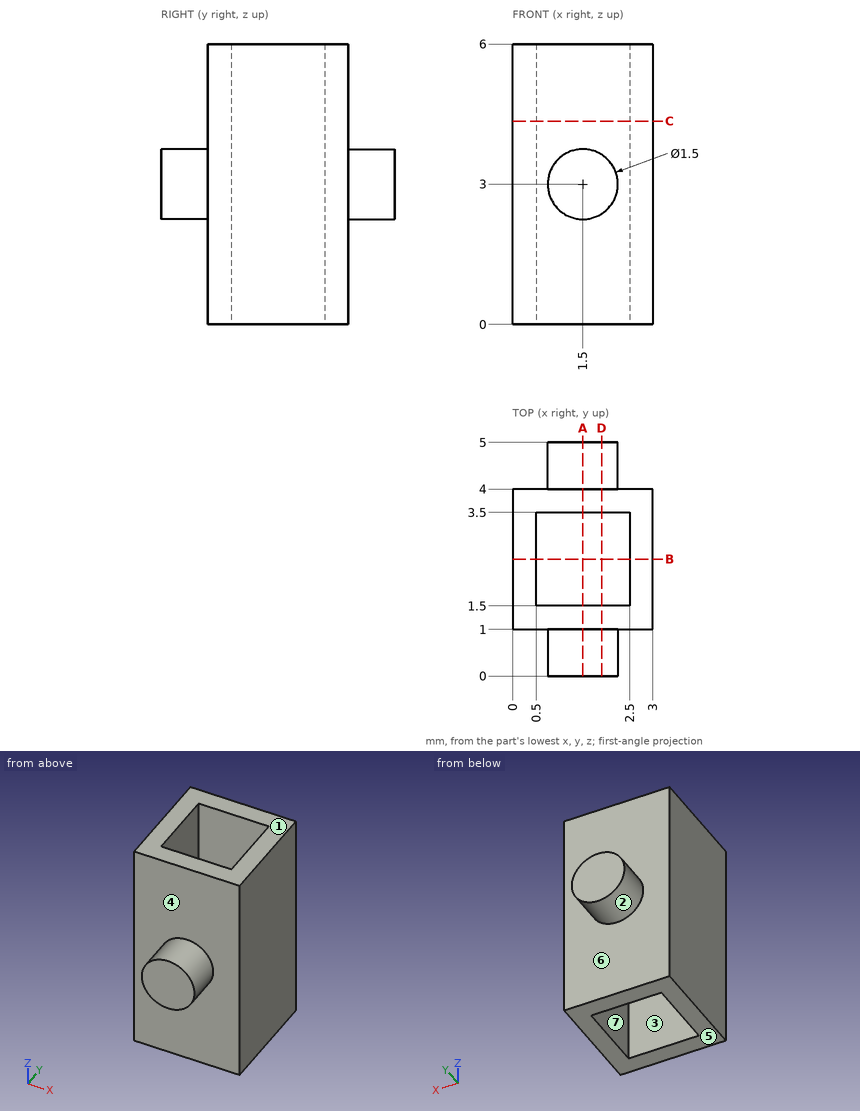
Geometry check sheet. Reference: drawing and pictorial views, mm from the part's lowest x, y, z. A direction names the side the tool comes from. Round coordinates to 2 decimals unless told otherwise and drop trailing zeros. Loops run counter-clockwise (first coordinate to the right, second up) from the corner with the lowest first, then second, coordinate; pieces in that order, holes last. Notation, with made-up numbers: (74.25, -25) - (91.25, -25) arc R19 cw to (91.25, -5) - close; hole circle Ø3 at (82, 44). An arc over 180 degrees is marked (long way). Use a Markdown table: item, result. Add a question column.
1. Section check C-C, the plane z = 4.35. Record the boundary of the cut face in (x, y), plus the area to 3 significant figures.
2. Thickness scan on probe 1 along Y at (x, z) = (1.9, 5.05); probe 2 along X at (y, z) = (3.15, 1.9); probe 3 along Y at (x, z) = (2.8, 2.9). Record the ranges inside material, lowest first. Write a range as [from, to].
3. Access from +Z, -Z, +X, -X, +Y, -Y to the whole of each face (thin tool, end or side, straight path). Record for the marked faces 1, 2, 3 and 4.
4. Section check D-D, the plane x = 1.9. Record the boundary of the cut face in (y, z).
5. Section check A-A, the plane x = 1.5. Record the boundary of the cut face in (y, z).
6. Release check for a two-part mould opening along Y. For the marked faces 5, 6 and 7 record: released by +Y, released by -Y, zero draft, split by the parting line, or undercut.
7. Section check B-B, the plane y = 2.5. Record the boundary of the cut face in (x, z).
Checks:
| question | item | result |
|---|---|---|
| 1 | outline | (0, 1) - (3, 1) - (3, 4) - (0, 4) - close; hole (0.5, 1.5) - (2.5, 1.5) - (2.5, 3.5) - (0.5, 3.5) - close |
| 1 | area | 5.00 mm^2 |
| 2 | probe 1 | y = [1, 1.5], [3.5, 4] |
| 2 | probe 2 | x = [0, 0.5], [2.5, 3] |
| 2 | probe 3 | y = [1, 4] |
| 3 | face 1 | +Z, +X, -X, +Y, -Y |
| 3 | face 2 | +Y |
| 3 | face 3 | +Z, -Z |
| 3 | face 4 | -Y |
| 4 | outline | (0, 2.37) - (1, 2.37) - (1, 0) - (1.5, 0) - (1.5, 6) - (1, 6) - (1, 3.63) - (0, 3.63) - close; (3.5, 0) - (4, 0) - (4, 2.37) - (5, 2.37) - (5, 3.63) - (4, 3.63) - (4, 6) - (3.5, 6) - close |
| 5 | outline | (0, 2.25) - (1, 2.25) - (1, 0) - (1.5, 0) - (1.5, 6) - (1, 6) - (1, 3.75) - (0, 3.75) - close; (3.5, 0) - (4, 0) - (4, 2.25) - (5, 2.25) - (5, 3.75) - (4, 3.75) - (4, 6) - (3.5, 6) - close |
| 6 | face 5 | zero draft |
| 6 | face 6 | released by +Y |
| 6 | face 7 | undercut |
| 7 | outline | (0, 0) - (0.5, 0) - (0.5, 6) - (0, 6) - close; (2.5, 0) - (3, 0) - (3, 6) - (2.5, 6) - close |
